from build123d import *

# Parameters (mm, degrees)
SKETCH_3_W          = 130
SKETCH_3_H          = 15
EXTRUDE_1_DEPTH     = 3
CUT_EXTRUDE_1_DEPTH = 35
SKETCH_5_W          = 3
SKETCH_5_H          = 15
EXTRUDE_2_DEPTH     = 50
SKETCH_6_R          = 2.5
CUT_EXTRUDE_2_DEPTH = 160


with BuildPart() as part:
    # 草图3 → 凸台-拉伸1 (new body)
    with BuildSketch(Plane(origin=(0, 0, 0), x_dir=(1, 0, 0), z_dir=(0, 1, 0))):
        Rectangle(SKETCH_3_W, SKETCH_3_H)
    extrude(amount=EXTRUDE_1_DEPTH)

    # 草图4 → 切除-拉伸1 (cut)
    with BuildSketch(Plane(origin=(0, 3, 0), x_dir=(1, 0, 0), z_dir=(0, 1, 0))):
        with BuildLine():
            Line((-40, 2.5), (-32, 2.5))
            ThreePointArc((-32, 2.5), (-29.5, 0), (-32, -2.5))
            Line((-32, -2.5), (-40, -2.5))
            ThreePointArc((-40, -2.5), (-42.5, 0), (-40, 2.5))
        make_face()
        with BuildLine():
            Line((40, -2.5), (32, -2.5))
            ThreePointArc((32, -2.5), (29.5, 0), (32, 2.5))
            Line((32, 2.5), (40, 2.5))
            ThreePointArc((40, 2.5), (42.5, 0), (40, -2.5))
        make_face()
    extrude(amount=-CUT_EXTRUDE_1_DEPTH, mode=Mode.SUBTRACT)

    # 草图5 → 凸台-拉伸2 (add)
    with BuildSketch(Plane(origin=(0, 3, 0), x_dir=(1, 0, 0), z_dir=(0, 1, 0))):
        with Locations((-63.5, 0)):
            Rectangle(SKETCH_5_W, SKETCH_5_H)
        with Locations((63.5, 0)):
            Rectangle(SKETCH_5_W, SKETCH_5_H)
    extrude(amount=EXTRUDE_2_DEPTH)

    # 草图6 → 切除-拉伸2 (cut)
    with BuildSketch(Plane.ZY.offset(65)):
        with Locations((0, 47)):
            Circle(SKETCH_6_R)
    extrude(amount=-CUT_EXTRUDE_2_DEPTH, mode=Mode.SUBTRACT)


solid = part.part
Here's how the part is built. I have some questions about the finished solid (model axes, mm). A direction names the side the tool comes from. Coordinates: 2 decimals unless noted, no trailing zeros. Order: outer loops, then holes, each group sorted by start corner. A loop starts at its lowest first (then second) coordinate and runs counter-clockwise, first axis right, second up. Notation, with made-up numbers: (-13, 5.5) - (1, 5.5) arc R14 ccw to (1, 20.5) - close; hole circle Ø9 at (-29, 35). An arc over 180 degrees is marked (long way). Use CSV: the item, a comma, the result in double quotes. Start each with the question number.
1. Suppose I cut it at A-A on y = 47. List the corners of the cut face in (x, z) for me, then the cut area to 3 significant figures.
2. Please list where these lines run through material, in increasing order: line 1 (X direction, y = 39.5, z = 2.25); line 2 (Y direction, x = -64.25, z = 0); line 3 (Y direction, x = 51, z = 0.5). Write a range as from..to.
3. Suppose I cut it at D-D on x = -54. List the corners of the cut face in (y, z) for me.
4. For faces 1 (the face through (36, 2, -2.5)), 2 (the face through (-62, 28, 0)), 3 (the face through (65, 26, 0)), which set-ups out of +Z, -Z, +X, -X, +Y, -Y let a thin tool reach every point of the face, with its end or its side?
5. If we mould it in two halves opening along Y, with no side actions, what happens to faces 4 (the face through (63.48, 44.56, -0.54)), 5 (the face through (63, 53, 0)), 6 (the face through (-36, 2, 2.5))? For each: +Y half, -Y half, draft (parallel to the pull), parting line (faces both ways), or undercut.
6. I'm going to push flat-ended pins straight in: pin 1 (4 mm diameter, centred on x = 35.5, z = -1.5, fed in from +Y); pin 2 (6 mm diameter, centred on y = 47, z = 0, fed in from +X). Where does each tip first touch, or does it pass through?
7. Suppose I cut it at B-B on z = 0. List the corners of the cut face in (x, y) for me.
8. Suppose I cut it at C-C on y = 19. List the corners of the cut face in (x, z) for me.
Output:
1,outline,"(-65, -7.5) - (-62, -7.5) - (-62, -2.5) - (-65, -2.5) - close; (-65, 2.5) - (-62, 2.5) - (-62, 7.5) - (-65, 7.5) - close; (62, -7.5) - (65, -7.5) - (65, -2.5) - (62, -2.5) - close; (62, 2.5) - (65, 2.5) - (65, 7.5) - (62, 7.5) - close"
1,area,"60.0 mm2"
2,line 1,"x = -65..-62, 62..65"
2,line 2,"y = 0..44.5, 49.5..53"
2,line 3,"y = 0..3"
3,outline,"(0, -7.5) - (3, -7.5) - (3, 7.5) - (0, 7.5) - close"
4,face 1,"+Y, -Y"
4,face 2,"+Z, -Z, +Y"
4,face 3,"+Z, -Z, +X, +Y, -Y"
5,face 4,"undercut"
5,face 5,"+Y half"
5,face 6,"draft"
6,pin 1,"stops at y = 3"
6,pin 2,"stops at x = 65"
7,outline,"(-65, 0) - (-42.5, 0) - (-42.5, 3) - (-62, 3) - (-62, 44.5) - (-65, 44.5) - close; (-65, 49.5) - (-62, 49.5) - (-62, 53) - (-65, 53) - close; (-29.5, 0) - (29.5, 0) - (29.5, 3) - (-29.5, 3) - close; (42.5, 0) - (65, 0) - (65, 44.5) - (62, 44.5) - (62, 3) - (42.5, 3) - close; (62, 49.5) - (65, 49.5) - (65, 53) - (62, 53) - close"
8,outline,"(-65, -7.5) - (-62, -7.5) - (-62, 7.5) - (-65, 7.5) - close; (62, -7.5) - (65, -7.5) - (65, 7.5) - (62, 7.5) - close"
